```python
from build123d import *

# Parameters (mm, degrees)
F0_W     = 50
F0_H     = 50
F0_W_2   = 400
F0_H_2   = 400
F1_DEPTH = 50
F2_W     = 50
F2_H     = 50
F3_DEPTH = 800


with BuildPart() as f1:
    # F0 (on Top) → F1 (new body)
    with BuildSketch(Plane.XY):
        with Locations((25, 475)):
            Rectangle(F0_W, F0_H)
        with Locations((250, 475)):
            Rectangle(F0_W_2, F0_H)
        with Locations((475, 475)):
            Rectangle(F0_W, F0_H)
        with Locations((475, 250)):
            Rectangle(F0_W, F0_H_2)
        with Locations((475, 25)):
            Rectangle(F0_W, F0_H)
        with Locations((250, 25)):
            Rectangle(F0_W_2, F0_H)
        with Locations((25, 25)):
            Rectangle(F0_W, F0_H)
        with Locations((25, 250)):
            Rectangle(F0_W, F0_H_2)
    extrude(amount=F1_DEPTH)

    # F2 (on face) → F3 (join)
    with BuildSketch(Plane.XY.offset(50)):
        with Locations((25, 475)):
            Rectangle(F2_W, F2_H)
        with Locations((475, 475)):
            Rectangle(F2_W, F2_H)
        with Locations((475, 25)):
            Rectangle(F2_W, F2_H)
        with Locations((25, 25)):
            Rectangle(F2_W, F2_H)
    extrude(amount=F3_DEPTH)


solid = f1.part
```
CAD build for the part. Positions are in the model's coordinates, mm. A direction names the side the tool comes from. Round coordinates to 2 decimals unless told otherwise and drop trailing zeros. Loops run counter-clockwise (first coordinate to the right, second up) from the corner with the lowest first, then second, coordinate; pieces in that order, holes last. Notation, with made-up numbers: M -15,84 L 20,84 A19 ccw 20,98 Z; hole C 31.25,68 d9. An arc over 180 degrees is marked long. Use a Markdown table: item, result. Add a question column.
(1) Pull direction X, two halves, no side cores. Call faces 1 (the face through (500, 45, 329)), 2 (the face through (50, 247, 25)), 3 (the face through (45, 500, 329)): +X half, -X half, draft (parallel to the pull), parting line (faces both ways), or undercut.
(2) Flat gauge pin, fed straight in: pin 1 (25 mm diameter, centred on x = 468.5, y = 165, fed in from +Z). Where does the tip first touch, or does it go through?
(3) Cut at A-A (z = 308). Give the cut face in (x, y).
(4) Cut at D-D (x = 468). Give the cut face in (y, z).
(5) Which spindle directions (+Z, -Z, +X, -X, +Y, -Y) get a long thin tool onto all of the face, cutting with end or side? Do faces 4 (the face through (50, 475, 444)), 5 (the face through (253, 50, 25)), 6 (the face through (475, 450, 444)), 7 (the face through (25, 475, 850)). Say none if no direction does.
(6) Drill centre lines: line 1 (Y direction, x = 46, z = 718.5); line 2 (Z direction, x = 450.5, y = 295.5). Where is each one in solid material? Low to high.
(7) Cut at B-B (y = 87). Give the cut face in (x, z), and give its area (3 significant figures).
Geometry says:
| question | item | result |
|---|---|---|
| 1 | face 1 | +X half |
| 1 | face 2 | undercut |
| 1 | face 3 | draft |
| 2 | pin 1 | stops at z = 50 |
| 3 | outline | M 0,0 L 50,0 L 50,50 L 0,50 Z; M 0,450 L 50,450 L 50,500 L 0,500 Z; M 450,0 L 500,0 L 500,50 L 450,50 Z; M 450,450 L 500,450 L 500,500 L 450,500 Z |
| 4 | outline | M 0,0 L 500,0 L 500,850 L 450,850 L 450,50 L 50,50 L 50,850 L 0,850 Z |
| 5 | face 4 | +Z, +Y, -Y |
| 5 | face 5 | +Z, -Z |
| 5 | face 6 | +Z, +X, -X |
| 5 | face 7 | +Z, +X, -X, +Y, -Y |
| 6 | line 1 | y = 0 to 50, 450 to 500 |
| 6 | line 2 | z = 0 to 50 |
| 7 | outline | M 0,0 L 50,0 L 50,50 L 0,50 Z; M 450,0 L 500,0 L 500,50 L 450,50 Z |
| 7 | area | 5,000 mm² |
